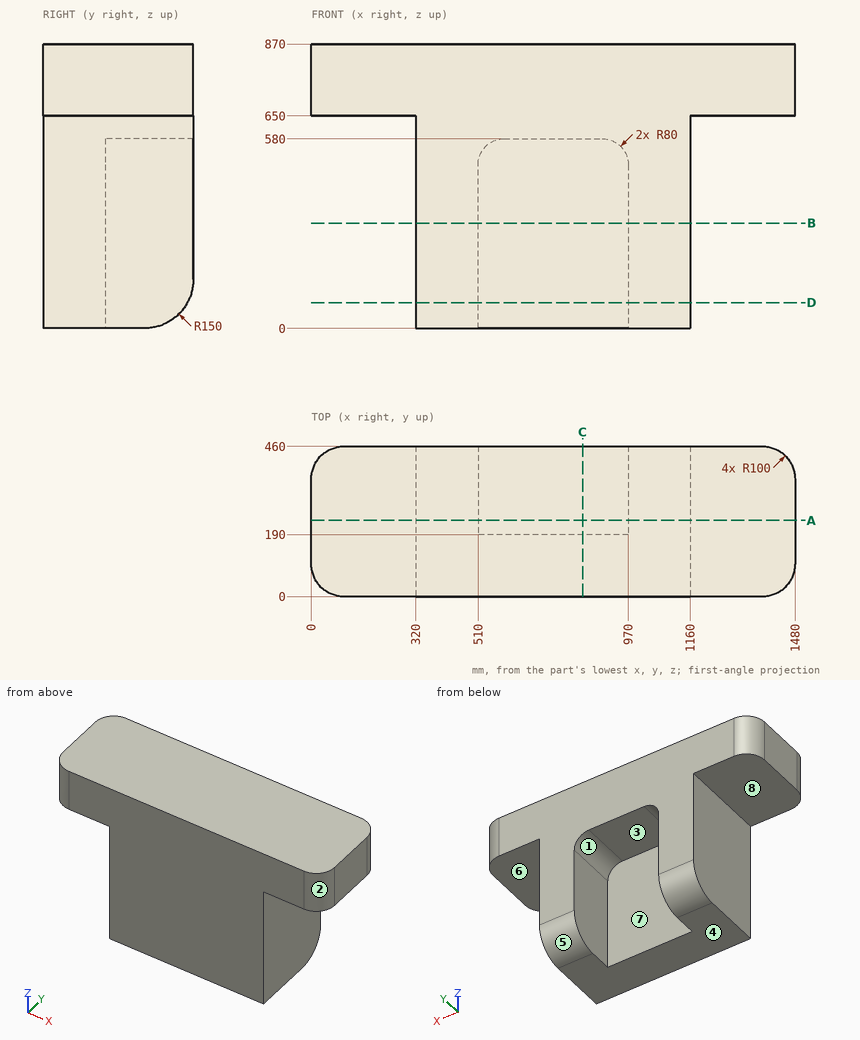
Drawing for the job (mm, zero at the part's lowest x, y, z). A direction names the side the tool comes from. Give positions to 0.01 mm unless a question says otherwise; leave off trailing zeros. Loops run counter-clockwise (first coordinate to the right, second up) from the corner with the lowest first, then second, coordinate; pieces in that order, holes last.
Item 1: Drill centre lines: line 1 along X through (y, z) = (251.5, 332.5); line 2 along Y through (x, z) = (789, 516); line 3 along X through (y, z) = (186, 458). Where is each one in solid material? Low to high.
Check values:
line 1: x = 320 to 510, 970 to 1160
line 2: y = 0 to 190
line 3: x = 320 to 1160
Item 2: Slice it at A-A (y = 233.5). Write the cut outline in (x, z), plus the area to 3 significant figures.
Check values:
outline: (0, 650) - (320, 650) - (320, 0) - (510, 0) - (510, 500) arc R80 cw to (590, 580) - (890, 580) arc R80 cw to (970, 500) - (970, 0) - (1160, 0) - (1160, 650) - (1480, 650) - (1480, 870) - (0, 870) - close
area: 608,000 mm2
Item 3: Mould opens along X. For the marked faces 1, 2, 3 and 4 say: +X half, -X half, draft (parallel to the pull), parting line (faces both ways), or undercut.
Check values:
face 1: undercut
face 2: +X half
face 3: undercut
face 4: draft
Item 4: Slice it at D-D (z = 78.5). Write the cut outline in (x, y), plus the area to 3 significant figures.
Check values:
outline: (320, 0) - (1160, 0) - (1160, 441.86) - (970, 441.86) - (970, 190) - (510, 190) - (510, 441.86) - (320, 441.86) - close
area: 255,000 mm2
Item 5: Slice it at C-C (x = 830). Write the cut outline in (y, z).
Check values:
outline: (0, 0) - (190, 0) - (190, 580) - (460, 580) - (460, 870) - (0, 870) - close
Item 6: Drop flat-ended pins along their axis: P1, Ø2, axis at y = 294.5, z = 496.5, coming from the +X side; P2, Ø8, axis at x = 850.5, z = 572, coming from the +Y side; P3, Ø6, axis at y = 267.5, z = 296, coming from the -X side. Give the stop position or say it passes through.
Check values:
P1: stops at x = 1160
P2: stops at y = 190
P3: stops at x = 320
Item 7: Which spindle directions (+Z, -Z, +X, -X, +Y, -Y) get a long thin tool onto all of the face, cutting with end or side? Do the marked faces 5, 6, 7 and 8. Say none if no direction does.
Check values:
face 5: -Z, +X, -X, +Y
face 6: -Z, +X, +Y, -Y
face 7: -Z, +Y
face 8: -Z, -X, +Y, -Y
Item 8: Slice it at B-B (z = 321.5). Write the cut outline in (x, y), plus the area to 3 significant figures.
Check values:
outline: (320, 0) - (1160, 0) - (1160, 460) - (970, 460) - (970, 190) - (510, 190) - (510, 460) - (320, 460) - close
area: 262,000 mm2
